Input: part model. Units: mm. Frame: model coordinates. A direction names the side the tool comes from. Round coordinates to 2 decimals unless told otherwise and drop trailing zeros. Loops run counter-clockwise (first coordinate to the right, second up) from the corner with the lowest first, then second, coordinate; pieces in that order, holes last. Notation, with made-up numbers: (-18.75, 7) -> (30.25, 7) arc R20 cw to (30.25, 17) -> close; hole circle Ø8 at (47.25, 52). An arc over 180 degrees is marked (long way). Answer as a JSON object with one key per item and string values.
```python
from build123d import *

# Parameters (mm, degrees)
SKETCH1_R           = 3
SKETCH1_W           = 25
SKETCH1_H           = 6
BOSS_EXTRUDE1_DEPTH = 6


with BuildPart() as part:
    # Sketch1 → Boss-Extrude1 (new body)
    with BuildSketch(Plane(origin=(0, 0, 0), x_dir=(1, 0, 0), z_dir=(0, 1, 0))):
        with BuildLine():
            Line((-10, 62.761766306), (10, 62.761766306))
            ThreePointArc((10, 62.761766306), (17.071067812, 59.832834118), (20, 52.761766306))
            Line((20, 52.761766306), (20, -57.238233694))
            Line((20, -57.238233694), (13, -57.238233694))
            Line((13, -57.238233694), (13, -63.238233694))
            Line((13, -63.238233694), (2, -63.238233694))
            Line((2, -63.238233694), (2, -55.238233694))
            Line((2, -55.238233694), (3.5, -55.238233694))
            Line((3.5, -55.238233694), (3.5, -52.038233694))
            Line((3.5, -52.038233694), (2, -52.038233694))
            Line((2, -52.038233694), (2, -48.038233694))
            Line((2, -48.038233694), (-2, -48.038233694))
            Line((-2, -48.038233694), (-2, -52.038233694))
            Line((-2, -52.038233694), (-3.5, -52.038233694))
            Line((-3.5, -52.038233694), (-3.5, -55.238233694))
            Line((-3.5, -55.238233694), (-2, -55.238233694))
            Line((-2, -55.238233694), (-2, -63.238233694))
            Line((-2, -63.238233694), (-13, -63.238233694))
            Line((-13, -63.238233694), (-13, -57.238233694))
            Line((-13, -57.238233694), (-20, -57.238233694))
            Line((-20, -57.238233694), (-20, 52.761766306))
            ThreePointArc((-20, 52.761766306), (-17.071067812, 59.832834118), (-10, 62.761766306))
        make_face()
        with Locations((0, 43.761766306)):
            Circle(SKETCH1_R, mode=Mode.SUBTRACT)
        with Locations((0, -1.238233694)):
            Rectangle(SKETCH1_W, SKETCH1_H, mode=Mode.SUBTRACT)
    extrude(amount=BOSS_EXTRUDE1_DEPTH)


solid = part.part
```
1) Reachability of faces 4 (the face through (0, 3, 4.238)), 5 (the face through (-13, 3, 60)), 6 (the face through (2, 3, 59)), 7 (the face through (0, 3, -62.762)), 8 (the face through (17, 3, 57.238)) from +Z, -Z, +X, -X, +Y, -Y: full face, straight path, thin tool, end or side. Return the list, or none.
Output:
{"face 4": "+Y, -Y", "face 5": "+Z, -X, +Y, -Y", "face 6": "+Z, +Y, -Y", "face 7": "-Z, +X, -X, +Y, -Y", "face 8": "+Z, +X, +Y, -Y"}
2) Ray query, probe 1 along Z at (x, y) = (0, 4.4); probe 2 along X at (y, z) = (1.5, -0.5); probe 3 along Z at (x, y) = (-6, 2). Return the intervals inside material, ascending.
Output:
{"probe 1": "z = -62.76 to -46.76, -40.76 to -1.76, 4.24 to 48.04", "probe 2": "x = -20 to -12.5, 12.5 to 20", "probe 3": "z = -62.76 to -1.76, 4.24 to 63.24"}
3) Section B-B, the plane x = 5. Output: boundary loops of the cut face in (y, z).
Output:
{"outline": "(0, -62.76) -> (6, -62.76) -> (6, -1.76) -> (0, -1.76) -> close; (0, 4.24) -> (6, 4.24) -> (6, 63.24) -> (0, 63.24) -> close"}
4) Contact query for flat-ended pins moving along their axis: P1, Ø3, axis at y = 3, z = 60.5, coming from the -X side; P2, Ø1, axis at x = 1, y = 1.5, coming from the +Z side; P3, Ø1.8, axis at y = 3.5, z = 59.5, coming from the +X side. Output: stop coordinate, or through.
Output:
{"P1": "stops at x = -13", "P2": "stops at z = 48.04", "P3": "stops at x = 13"}
5) Section A-A, the plane x = 0. Output: boundary loops of the cut face in (y, z), plus the area to 3 significant figures.
Output:
{"outline": "(0, -62.76) -> (6, -62.76) -> (6, -46.76) -> (0, -46.76) -> close; (0, -40.76) -> (6, -40.76) -> (6, -1.76) -> (0, -1.76) -> close; (0, 4.24) -> (6, 4.24) -> (6, 48.04) -> (0, 48.04) -> close", "area": "593 mm^2"}
6) Section C-C, the plane y = 1.25. Output: boundary loops of the cut face in (x, z).
Output:
{"outline": "(-20, -52.76) arc R10 ccw to (-10, -62.76) -> (10, -62.76) arc R10 ccw to (20, -52.76) -> (20, 57.24) -> (13, 57.24) -> (13, 63.24) -> (2, 63.24) -> (2, 55.24) -> (3.5, 55.24) -> (3.5, 52.04) -> (2, 52.04) -> (2, 48.04) -> (-2, 48.04) -> (-2, 52.04) -> (-3.5, 52.04) -> (-3.5, 55.24) -> (-2, 55.24) -> (-2, 63.24) -> (-13, 63.24) -> (-13, 57.24) -> (-20, 57.24) -> close; hole (-12.5, -1.76) -> (12.5, -1.76) -> (12.5, 4.24) -> (-12.5, 4.24) -> close; hole circle Ø6 at (0, -43.76)"}
7) Draft query along X for faces 1 (the face through (14, 0, -1)), 2 (the face through (-20, 3, 3)), 3 (the face through (-2, 3, 59)). Return one class per face: +X half, -X half, draft (parallel to the pull), parting line (faces both ways), or undercut.
Output:
{"face 1": "draft", "face 2": "-X half", "face 3": "undercut"}
